For this review, take the finished solid that the model builds, in its own axes (mm). Round coordinates to 2 decimals unless told otherwise and drop trailing zeros. Loops run counter-clockwise (first coordinate to the right, second up) from the corner with the lowest first, then second, coordinate; pieces in that order, holes last.
1) Take a section at A-A (x = 0). State the section outline as (y, z) points (1 decimal), then the cut area to 3 significant figures.
2) Take a section at B-B (y = 7.5). State the section outline as (x, z) points (1 decimal).
3) Wall thickness on L1, parallel to X at y = 0.5, z = 1.25; L2, parallel to Y at x = 24, z = 1.05; L3, parallel to Y at x = 20.5, z = 1.35: over which ranges is each line inside the solid? List them lowest first.
4) Take a section at D-D (z = 2.1). Give the number of separate pieces and of enclosed holes in the cut face, then the cut area to 3 significant figures.
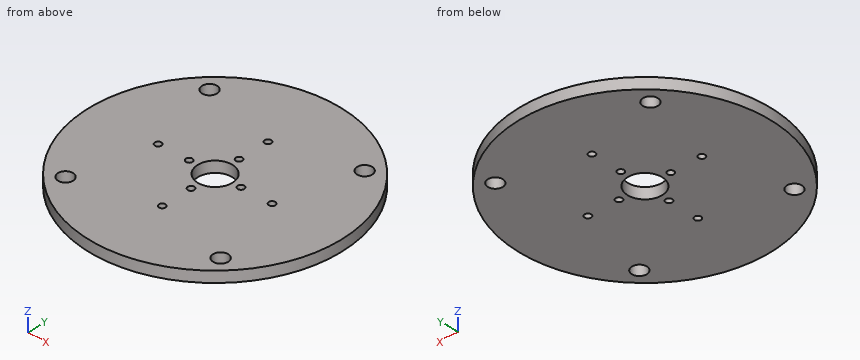
Autodesk Fusion 360 part; units mm, degrees
sketch "Sketch1" plane through (0, 0, 0) normal (0, 0, 1) x (1, 0, 0)
  circle A0 centre (0, 0) radius 7.5
  circle A1 centre (16.5, 0) radius 0.9375
  circle A2 centre (-16.5, 0) radius 0.9375
  circle A3 centre (0, -16.5) radius 0.9375
  circle A4 centre (0, 16.5) radius 0.9375
  line L0 (0, 0) -> (18.2563, 0) construction
  circle A5 centre (22.4506, 22.4506) radius 2.159
  circle A6 centre (22.4506, -22.4506) radius 2.159
  circle A7 centre (-22.4506, -22.4506) radius 2.159
  circle A8 centre (-22.4506, 22.4506) radius 2.159
  circle A9 centre (0, 0) radius 5
  circle A10 centre (0, 0) radius 36.5125
  line L1 (0, 0) -> (22.4506, 22.4506)
  line L2 (0, 0) -> (21.082, 0) construction
  line L3 (0, 0) -> (22.4506, -22.4506)
  line L4 (0, 0) -> (21.082, 0) construction
  line L5 (0, 0) -> (-22.4506, -22.4506)
  line L6 (0, 0) -> (21.082, 0) construction
  line L7 (0, 0) -> (-22.4506, 22.4506)
  line L8 (0, 0) -> (21.082, 0) construction
  arc A11 (-20.873, 23.9245) -> (20.873, 23.9245) centre (0, 0) ccw
  line L9 (16.5, 0) -> (10.5, 0)
  circle A12 centre (0, 0) radius 5.2451
  circle A13 centre (7.5, 0) radius 0.9375
  circle A14 centre (0, 7.5) radius 0.9375
  circle A15 centre (-7.5, 0) radius 0.9375
  circle A16 centre (0, -7.5) radius 0.9375
  dimension "d2" = 15
  dimension "d6" = 1.875
  dimension "d7" = 1.875
  dimension "d8" = 1.875
  dimension "d9" = 1.875
  dimension "d16" = 4.318
  dimension "d17" = 4.318
  dimension "d18" = 4.318
  dimension "d19" = 4.318
  dimension "d21" = 10
  dimension "d24" = 73.025
  dimension "d25" = 63.5
  dimension "d26" = 45
  dimension "d27" = 45
  dimension "d28" = 135
  dimension "d29" = 135
  dimension "d31" = 6
  dimension "d32" = 10.4902
  dimension "d33" = 1.875
  dimension "d35" = 360
extrude "Extrude1" add sketch "Sketch1" along normal blind 3.175 contours A0 L1 L3 A12 A13 | A0 A5 A6 L1 L3 A11 A13 | A0 L1 L7 A12 A14 | A0 A6 A7 L3 L5 A11 A16 | A0 L3 L5 A12 A16 | A9 L1 L3 A12 | A9 L1 L7 A12 | A9 L3 L5 A12 | A0 L5 L7 A12 A15 | A9 L5 L7 A12 | A0 A7 A8 L5 L7 A11 A15 | A10
equation "d22 = ( 1 / 8 ) * 1 in"
Response:
1. outline: (-36.5, 0) - (-17.4, 0) - (-17.4, 3.2) - (-36.5, 3.2) - close; (-15.6, 0) - (-8.4, 0) - (-8.4, 3.2) - (-15.6, 3.2) - close; (-6.6, 0) - (-5, 0) - (-5, 3.2) - (-6.6, 3.2) - close; (5, 0) - (6.6, 0) - (6.6, 3.2) - (5, 3.2) - close; (8.4, 0) - (15.6, 0) - (15.6, 3.2) - (8.4, 3.2) - close; (17.4, 0) - (36.5, 0) - (36.5, 3.2) - (17.4, 3.2) - close
1. area: 176 mm2
2. outline: (-35.7, 0) - (-0.9, 0) - (-0.9, 3.2) - (-35.7, 3.2) - close; (0.9, 0) - (35.7, 0) - (35.7, 3.2) - (0.9, 3.2) - close
3. L1: x = -36.51 to -17.29, -15.71 to -8.29, -6.71 to -4.97, 4.97 to 6.71, 8.29 to 15.71, 17.29 to 36.51
3. L2: y = -27.52 to -23.95, -20.95 to 20.95, 23.95 to 27.52
3. L3: y = -30.21 to -23.38, -21.53 to 21.53, 23.38 to 30.21
4. separate pieces: 1
4. enclosed holes: 13
4. area: 4,030 mm2
